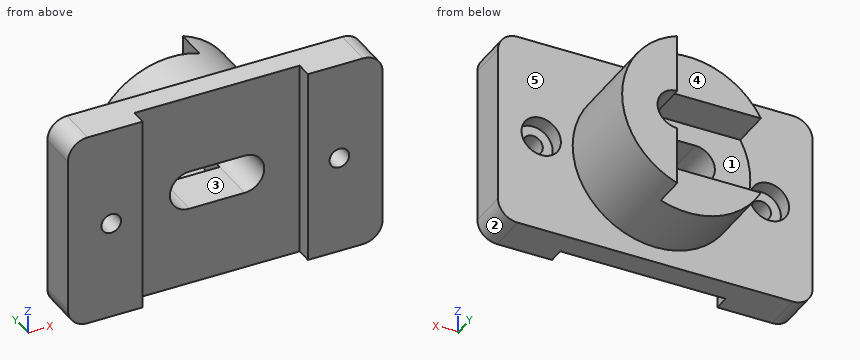
from build123d import *

# Parameters (mm, degrees)
EXTRUDE_1_DEPTH          = 10
SKETCH_2_R               = 21
EXTRUDE_2_DEPTH          = 34
CUT_EXTRUDE_1_DEPTH      = 35
CUT_EXTRUDE_2_DEPTH      = 8
CUT_EXTRUDE_3_DEPTH      = 10
SKETCH_6_R               = 5
CUT_EXTRUDE_4_DEPTH      = 4
SKETCH_7_R               = 2.5
CUT_EXTRUDE_5_DEPTH      = 7
SKETCH_8_W               = 42
SKETCH_8_H               = 4
CUT_EXTRUDE_6_DEPTH      = 26
CUT_EXTRUDE_6_DEPTH_BACK = 26


with BuildPart() as part:
    # 草图1 → 凸台-拉伸1 (new body)
    with BuildSketch(Plane(origin=(0, 0, 0), x_dir=(1, 0, 0), z_dir=(0, 1, 0))):
        with BuildLine():
            Line((-35, 25), (35, 25))
            ThreePointArc((35, 25), (38.535533906, 23.535533906), (40, 20))
            Line((40, 20), (40, -20))
            ThreePointArc((40, -20), (38.535533906, -23.535533906), (35, -25))
            Line((35, -25), (-35, -25))
            ThreePointArc((-35, -25), (-38.535533906, -23.535533906), (-40, -20))
            Line((-40, -20), (-40, 20))
            ThreePointArc((-40, 20), (-38.535533906, 23.535533906), (-35, 25))
        make_face()
    extrude(amount=EXTRUDE_1_DEPTH)

    # 草图2 → 凸台-拉伸2 (add)
    with BuildSketch(Plane(origin=(0, 0, 0), x_dir=(1, 0, 0), z_dir=(0, 1, 0))):
        Circle(SKETCH_2_R)
    extrude(amount=EXTRUDE_2_DEPTH)

    # 草图3 → 切除-拉伸1 (cut, through all)
    with BuildSketch(Plane(origin=(0, 34, 0), x_dir=(1, 0, 0), z_dir=(0, 1, 0))):
        with BuildLine():
            Line((-7, 5), (7, 5))
            ThreePointArc((7, 5), (12, 0), (7, -5))
            Line((7, -5), (-7, -5))
            ThreePointArc((-7, -5), (-12, 0), (-7, 5))
        make_face()
    extrude(amount=-CUT_EXTRUDE_1_DEPTH, mode=Mode.SUBTRACT)

    # 草图4 → 切除-拉伸2 (cut)
    with BuildSketch(Plane(origin=(0, 34, 0), x_dir=(1, 0, 0), z_dir=(0, 1, 0))):
        with BuildLine():
            Line((7, 19.798989873), (7, -19.798989873))
            ThreePointArc((7, -19.798989873), (-21, 0), (7, 19.798989873))
        make_face()
    extrude(amount=-CUT_EXTRUDE_2_DEPTH, mode=Mode.SUBTRACT)

    # 草图5 → 切除-拉伸3 (cut)
    with BuildSketch(Plane(origin=(0, 26, 0), x_dir=(1, 0, 0), z_dir=(0, 1, 0))):
        with BuildLine():
            Line((-18.466185313, 10), (7, 10))
            Line((7, 10), (7, -10))
            Line((7, -10), (-18.466185313, -10))
            ThreePointArc((-18.466185313, -10), (-21, 0), (-18.466185313, 10))
        make_face()
    extrude(amount=-CUT_EXTRUDE_3_DEPTH, mode=Mode.SUBTRACT)

    # 草图6 → 切除-拉伸4 (cut)
    with BuildSketch(Plane(origin=(0, 10, 0), x_dir=(1, 0, 0), z_dir=(0, 1, 0))):
        with Locations((-29, 0)):
            Circle(SKETCH_6_R)
    cut_extrude_4 = extrude(amount=-CUT_EXTRUDE_4_DEPTH, mode=Mode.SUBTRACT)

    # 草图7 → 切除-拉伸5 (cut, through all)
    with BuildSketch(Plane(origin=(0, 6, 0), x_dir=(1, 0, 0), z_dir=(0, 1, 0))):
        with Locations((-29, 0)):
            Circle(SKETCH_7_R)
    cut_extrude_5 = extrude(amount=-CUT_EXTRUDE_5_DEPTH, mode=Mode.SUBTRACT)

    # 镜向1: 切除-拉伸4, 切除-拉伸5 across plane
    add(cut_extrude_4.mirror(Plane(origin=(0, 0, 0), x_dir=(0, 0, 1), z_dir=(1, 0, 0))), mode=Mode.SUBTRACT)
    add(cut_extrude_5.mirror(Plane(origin=(0, 0, 0), x_dir=(0, 0, 1), z_dir=(1, 0, 0))), mode=Mode.SUBTRACT)

    # 草图8 → 切除-拉伸6 (cut, two sides)
    with BuildSketch(Plane.XY) as cut_extrude_6_sk:
        with Locations((0, 2)):
            Rectangle(SKETCH_8_W, SKETCH_8_H)
    extrude(amount=CUT_EXTRUDE_6_DEPTH, mode=Mode.SUBTRACT)
    extrude(cut_extrude_6_sk.sketch, amount=-CUT_EXTRUDE_6_DEPTH_BACK, mode=Mode.SUBTRACT)


solid = part.part
Input: part model. Units: mm. Frame: model coordinates. Face numbers are marked on the shaded views. A direction names the side the tool comes from. Round coordinates to 2 decimals unless told otherwise and drop trailing zeros. Write each loop counter-clockwise with the first axis right and the second up, starting at its lowest first coordinate (ties: lowest second). Pieces come first, ordered by that corner, then holes.
1) Contact query for flat-ended pins moving along their axis: P1, Ø5.5, axis at x = 0, z = -16.5, coming from the +Y side; P2, Ø8, axis at x = 5.5, z = -2, coming from the +Y side; P3, Ø5, axis at x = -2, y = 17, coming from the +Z side; P4, Ø1, axis at y = 27.5, z = -0.5, coming from the -X side. Output: stop coordinate, or through.
2) Reachability of the marked faces 1, 2, 3, 4 and 5 from +Z, -Z, +X, -X, +Y, -Y: full face, straight path, thin tool, end or side. Return the list, or none.
3) Cut plane C-C (y = 8). Return the cut outline in (x, z).
4) Cut plane B-B (z = 0). Count the separate pieces of the cut face and the enclosed holes in it, then the cut area to 3 significant figures.
5) Ray query, L1, parallel to X at y = 2.3, z = 0; L2, parallel to X at y = 7.5, z = 0; L3, parallel to Z at x = 29, y = 2. Return the intervals inside material, ascending.
6) Cut plane D-D (y = 20). Return the cut outline in (x, z).
7) Cut plane A-A (x = -29). Return the cut outline in (y, z).
Geometry says:
1. P1: stops at y = 26
1. P2: stops at y = 34
1. P3: stops at z = 21
1. P4: stops at x = 11.9
2. face 1: -X, +Y
2. face 2: -Z, +X, +Y, -Y
2. face 3: +Y, -Y
2. face 4: +Z, -Z, -X, +Y
2. face 5: +Y
3. outline: (-40, -20) arc R5 ccw to (-35, -25) - (35, -25) arc R5 ccw to (40, -20) - (40, 20) arc R5 ccw to (35, 25) - (-35, 25) arc R5 ccw to (-40, 20) - close; hole circle Ø10 at (-29, 0); hole (-7, -5) - (7, -5) arc R5 ccw to (7, 5) - (-7, 5) arc R5 ccw to start; hole circle Ø10 at (29, 0)
4. separate pieces: 4
4. enclosed holes: 0
4. area: 618 mm2
5. L1: x = -40 to -31.5, -26.5 to -21, 21 to 26.5, 31.5 to 40
5. L2: x = -40 to -34, -24 to -12, 12 to 24, 34 to 40
5. L3: z = -25 to -2.5, 2.5 to 25
6. outline: (-18.47, -10) arc R21 ccw (long way) to (-18.47, 10) - (7, 10) - (7, 5) arc R5 cw to (7, -5) - (7, -10) - close
7. outline: (0, -25) - (10, -25) - (10, -5) - (6, -5) - (6, -2.5) - (0, -2.5) - close; (0, 2.5) - (6, 2.5) - (6, 5) - (10, 5) - (10, 25) - (0, 25) - close
